Input: dimensioned drawing with shaded views. Units: mm. Origin: part minimum x, y, z. A direction names the side the tool comes from. Coordinates: 2 decimals unless noted, no trailing zeros. Order: outer loops, then holes, each group sorted by start corner. A loop starts at its lowest first (then second) coordinate and runs counter-clockwise, first axis right, second up. Notation, with made-up numbers: M 8.25,52 L 67.25,52 A20 cw 67.25,65 Z; hole C -23,-23 d6. An arc over 180 degrees is marked long. Use CSV: the item, a comma, the result in double quotes. Start each with the question number.
1. Material intervals for line 1 (X direction, y = 86.5, z = 9.5); line 2 (X direction, y = 92.5, z = 175); line 3 (Z direction, x = 19, y = 59), sorted ascending.
2. Section query A-A on y = 65.5. Return the cut outline in (x, z), and give its area (3 significant figures).
3. First-contact query: P1, Ø5, axis at x = 24, y = 105.5, coming from the +Z side; P2, Ø8, axis at x = 24.5, y = 108.5, coming from the -Z side; P3, Ø15.5, axis at y = 45, z = 146.5, coming from the +X side. Flat tips, straight axial feed; report the tip coordinate or a pass-through.
4. Section query B-B on x = 3.75. Return the cut outline in (y, z).
5. Section query C-C on z = 38.5. Return the cut outline in (x, y).
6. Section query D-D on y = 96. Return the cut outline in (x, z).
7. Set-up query: the marked faces 1 and 2. Return all of +Z, -Z, +X, -X, +Y, -Y with unobstructed straight access to the full face (end or side cutting, diameter ignored); none if empty.
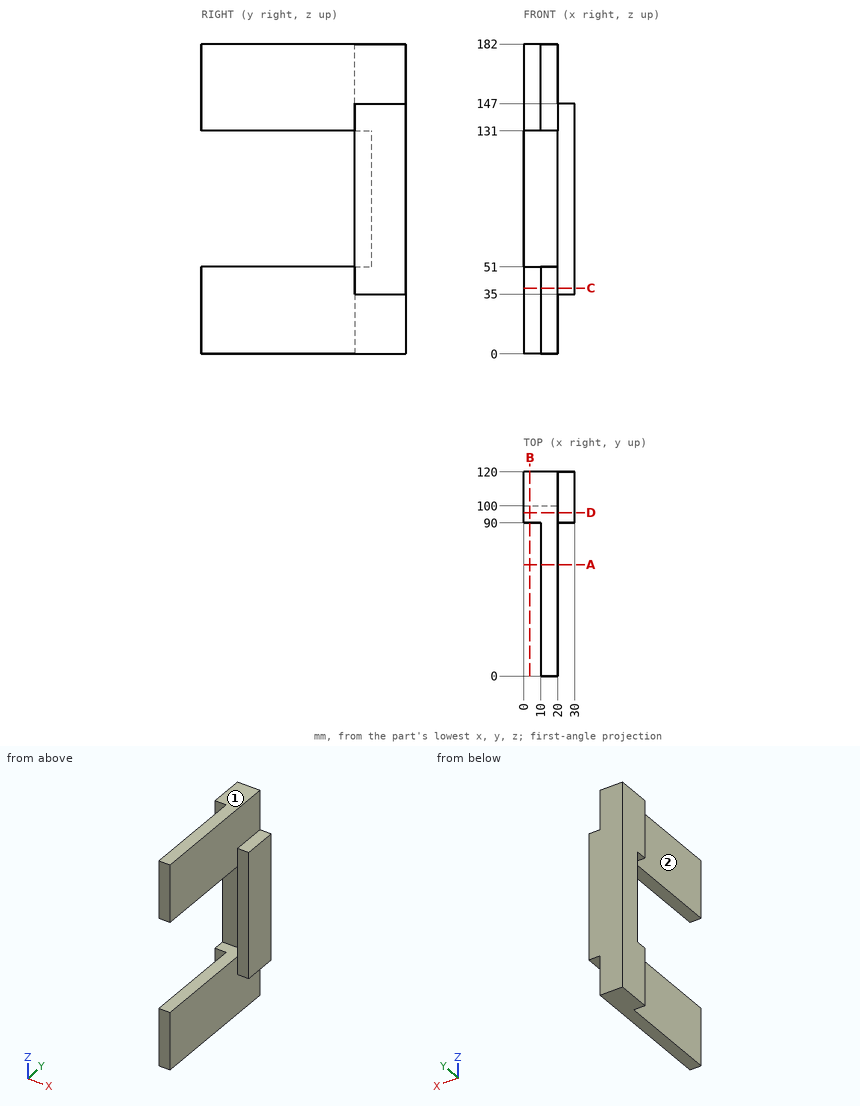
Results list:
1,line 1,"x = 10 to 20"
1,line 2,"x = 0 to 20"
1,line 3,"z = 0 to 51, 131 to 182"
2,outline,"M 10,0 L 20,0 L 20,51 L 10,51 Z; M 10,131 L 20,131 L 20,182 L 10,182 Z"
2,area,"1,020 mm²"
3,P1,"stops at z = 147"
3,P2,"stops at z = 35"
3,P3,"stops at x = 20"
4,outline,"M 90,0 L 120,0 L 120,182 L 90,182 L 90,131 L 100,131 L 100,51 L 90,51 Z"
5,outline,"M 0,90 L 10,90 L 10,0 L 20,0 L 20,90 L 30,90 L 30,120 L 0,120 Z"
6,outline,"M 0,0 L 20,0 L 20,35 L 30,35 L 30,147 L 20,147 L 20,182 L 0,182 L 0,131 L 20,131 L 20,51 L 0,51 Z"
7,face 1,"+Z, +X, -X, +Y, -Y"
7,face 2,"+Z, -Z, -X, -Y"
